```python
from build123d import *

# Parameters (mm, degrees)
SKETCH1_W                  = 84.6
SKETCH1_H                  = 55.3
BOSS_EXTRUDE1_DEPTH        = 2.4
SKETCH2_W                  = 82
SKETCH2_H                  = 54.2
BOSS_EXTRUDE2_DEPTH        = 1.1
SKETCH3_R                  = 0.5
BOSS_EXTRUDE3_DEPTH        = 0.8
CUT_EXTRUDE1_DEPTH         = 1
SKETCH5_W                  = 57
SKETCH5_H                  = 2.4
CUT_EXTRUDE2_DEPTH         = 0.2
SKETCH6_W                  = 45.3
SKETCH6_H                  = 2.4
CUT_EXTRUDE3_DEPTH         = 0.2
SKETCH7_W                  = 44.6
SKETCH7_H                  = 3
BOSS_EXTRUDE4_DEPTH        = 0.15
SKETCH8_W                  = 0.6
SKETCH8_H                  = 12.5
CUT_EXTRUDE4_DEPTH         = 1
SKETCH9_W                  = 4
SKETCH9_H                  = 0.5
BOSS_EXTRUDE5_DEPTH        = 0.2
CHAMFER1_SIZE              = 0.2
CHAMFER1_SIZE_2            = 0.549495484
CHAMFER1_OF_MIRROR4_SIZE   = 0.2
CHAMFER1_OF_MIRROR4_SIZE_2 = 0.549495484
SKETCH10_W                 = 36
SKETCH10_H                 = 1.5
CUT_EXTRUDE5_DEPTH         = 10
BOSS_EXTRUDE7_DEPTH        = 12.5
BOSS_EXTRUDE7_DEPTH_BACK   = 12.5


with BuildPart() as part:
    # Sketch1 → Boss-Extrude1 (new body)
    with BuildSketch(Plane(origin=(0, 0, 0), x_dir=(1, 0, 0), z_dir=(0, 1, 0))):
        Rectangle(SKETCH1_W, SKETCH1_H)
    extrude(amount=-BOSS_EXTRUDE1_DEPTH)

    # Sketch2 → Boss-Extrude2 (add)
    with BuildSketch(Plane(origin=(0, 0, 0), x_dir=(1, 0, 0), z_dir=(0, 1, 0))):
        Rectangle(SKETCH2_W, SKETCH2_H)
    extrude(amount=BOSS_EXTRUDE2_DEPTH)

    # Sketch3 → Boss-Extrude3 (add)
    with BuildSketch(Plane.XZ.offset(2.4)):
        with Locations(Location((-41.8, 27.15, 0), (0, 0, 90))):
            Circle(SKETCH3_R)
        with Locations(Location((41.8, 27.15, 0), (0, 0, 90))):
            Circle(SKETCH3_R)
        with Locations(Location((41.8, -27.15, 0), (0, 0, 270))):
            Circle(SKETCH3_R)
        with Locations(Location((-41.8, -27.15, 0), (0, 0, 270))):
            Circle(SKETCH3_R)
    extrude(amount=BOSS_EXTRUDE3_DEPTH)

    # Sketch4 → Cut-Extrude1 (cut)
    with BuildSketch(Plane.XZ.offset(2.4)):
        with BuildLine():
            Line((-39.7, -22.4), (-41.3, -22.4))
            ThreePointArc((-41.3, -22.4), (-41.724264069, -22.224264069), (-41.9, -21.8))
            Line((-41.9, -21.8), (-41.9, 21.8))
            ThreePointArc((-41.9, 21.8), (-41.724264069, 22.224264069), (-41.3, 22.4))
            Line((-41.3, 22.4), (-39.7, 22.4))
            ThreePointArc((-39.7, 22.4), (-39.275735931, 22.224264069), (-39.1, 21.8))
            Line((-39.1, 21.8), (-39.1, -21.8))
            ThreePointArc((-39.1, -21.8), (-39.275735931, -22.224264069), (-39.7, -22.4))
        make_face()
    extrude(amount=-CUT_EXTRUDE1_DEPTH, mode=Mode.SUBTRACT)

    # Sketch5 → Cut-Extrude2 (cut)
    with BuildSketch(Plane.XY.offset(27.65)):
        with Locations((8.8, -1.2)):
            Rectangle(SKETCH5_W, SKETCH5_H)
    cut_extrude2 = extrude(amount=-CUT_EXTRUDE2_DEPTH, mode=Mode.SUBTRACT)

    # Mirror1: Cut-Extrude2 across plane
    add(cut_extrude2.mirror(Plane.XY), mode=Mode.SUBTRACT)

    # Sketch6 → Cut-Extrude3 (cut)
    with BuildSketch(Plane(origin=(42.3, 0, 0), x_dir=(0, 0, -1), z_dir=(1, 0, 0))):
        with Locations((0, -1.2)):
            Rectangle(SKETCH6_W, SKETCH6_H)
    extrude(amount=-CUT_EXTRUDE3_DEPTH, mode=Mode.SUBTRACT)

    # Sketch7 → Boss-Extrude4 (add)
    with BuildSketch(Plane.XZ.offset(2.4)):
        with Locations((15, 25.85)):
            Rectangle(SKETCH7_W, SKETCH7_H)
    boss_extrude4 = extrude(amount=BOSS_EXTRUDE4_DEPTH)

    # Mirror2: Boss-Extrude4 across plane
    add(boss_extrude4.mirror(Plane.XY))

    # Sketch8 → Cut-Extrude4 (cut)
    with BuildSketch(Plane(origin=(0, 0, 0), x_dir=(1, 0, 0), z_dir=(0, 1, 0))):
        with Locations((41.3, 0)):
            Rectangle(SKETCH8_W, SKETCH8_H)
    extrude(amount=-CUT_EXTRUDE4_DEPTH, mode=Mode.SUBTRACT)

    # Sketch9 → Boss-Extrude5 (add)
    with BuildSketch(Plane.XY.offset(27.45)):
        with Locations((-1.7, -1.2)):
            Rectangle(SKETCH9_W, SKETCH9_H)
        with Locations((26.3, -1.2)):
            Rectangle(SKETCH9_W, SKETCH9_H)
    boss_extrude5 = extrude(amount=BOSS_EXTRUDE5_DEPTH)

    # Chamfer1
    # the kernel refuses this chamfer: 0.549495484, 0.2 mm, written as the material it takes off along each edge
    with BuildSketch(Plane(origin=(29.72549829, -1.45, 27.65), x_dir=(0, -0.0990409022520511, -0.9950833631817485), z_dir=(-1, 0, 0))) as chamfer1_piece_1_section:
        Polygon((CHAMFER1_SIZE * 0.995083363182, -CHAMFER1_SIZE * 0.0990409022521), (-CHAMFER1_SIZE_2 * 0.0990409022324, -CHAMFER1_SIZE_2 * 0.995083362984), (0, 0), align=None)
    chamfer1_piece_1 = extrude(amount=6.85099658, mode=Mode.PRIVATE)
    chamfer1_piece_1 = split(chamfer1_piece_1, bisect_by=Plane(origin=(26.3, -1.261493049, 27.45), z_dir=(0, 0, 1)), keep=Keep.TOP, mode=Mode.PRIVATE)
    add(chamfer1_piece_1, mode=Mode.SUBTRACT)
    with BuildSketch(Plane(origin=(1.72549829, -1.45, 27.65), x_dir=(0, -0.0990409022520511, -0.9950833631817485), z_dir=(-1, 0, 0))) as chamfer1_piece_2_section:
        Polygon((CHAMFER1_SIZE * 0.995083363182, -CHAMFER1_SIZE * 0.0990409022521), (-CHAMFER1_SIZE_2 * 0.0990409022324, -CHAMFER1_SIZE_2 * 0.995083362984), (0, 0), align=None)
    chamfer1_piece_2 = extrude(amount=6.85099658, mode=Mode.PRIVATE)
    chamfer1_piece_2 = split(chamfer1_piece_2, bisect_by=Plane(origin=(-1.7, -1.261493049, 27.45), z_dir=(0, 0, 1)), keep=Keep.TOP, mode=Mode.PRIVATE)
    add(chamfer1_piece_2, mode=Mode.SUBTRACT)

    # Mirror4: Boss-Extrude5 across plane
    add(boss_extrude5.mirror(Plane.XY))

    # Chamfer1 of Mirror4
    # the kernel refuses this chamfer: 0.549495484, 0.2 mm, written as the material it takes off along each edge
    with BuildSketch(Plane(origin=(29.72549829, -1.45, -27.65), x_dir=(0, -0.0990409022520511, 0.9950833631817485), z_dir=(-1, 0, 0))) as chamfer1_of_mirror4_piece_1_section:
        Polygon((CHAMFER1_OF_MIRROR4_SIZE * 0.995083363182, CHAMFER1_OF_MIRROR4_SIZE * 0.0990409022521), (-CHAMFER1_OF_MIRROR4_SIZE_2 * 0.0990409022324, CHAMFER1_OF_MIRROR4_SIZE_2 * 0.995083362984), (0, 0), align=None)
    chamfer1_of_mirror4_piece_1 = extrude(amount=6.85099658, mode=Mode.PRIVATE)
    chamfer1_of_mirror4_piece_1 = split(chamfer1_of_mirror4_piece_1, bisect_by=Plane(origin=(26.3, -1.261493049, -27.45), z_dir=(0, 0, -1)), keep=Keep.TOP, mode=Mode.PRIVATE)
    add(chamfer1_of_mirror4_piece_1, mode=Mode.SUBTRACT)
    with BuildSketch(Plane(origin=(1.72549829, -1.45, -27.65), x_dir=(0, -0.0990409022520511, 0.9950833631817485), z_dir=(-1, 0, 0))) as chamfer1_of_mirror4_piece_2_section:
        Polygon((CHAMFER1_OF_MIRROR4_SIZE * 0.995083363182, CHAMFER1_OF_MIRROR4_SIZE * 0.0990409022521), (-CHAMFER1_OF_MIRROR4_SIZE_2 * 0.0990409022324, CHAMFER1_OF_MIRROR4_SIZE_2 * 0.995083362984), (0, 0), align=None)
    chamfer1_of_mirror4_piece_2 = extrude(amount=6.85099658, mode=Mode.PRIVATE)
    chamfer1_of_mirror4_piece_2 = split(chamfer1_of_mirror4_piece_2, bisect_by=Plane(origin=(-1.7, -1.261493049, -27.45), z_dir=(0, 0, -1)), keep=Keep.TOP, mode=Mode.PRIVATE)
    add(chamfer1_of_mirror4_piece_2, mode=Mode.SUBTRACT)

    # Sketch10 → Cut-Extrude5 (cut)
    with BuildSketch(Plane.ZY.offset(42.3)):
        with Locations((0, -0.75)):
            Rectangle(SKETCH10_W, SKETCH10_H)
    extrude(amount=-CUT_EXTRUDE5_DEPTH, mode=Mode.SUBTRACT)

    # Sketch13 → Boss-Extrude7 (add, two sides: drawn at the far end of the back side and taken through both)
    with BuildSketch(Plane.XY.offset(-BOSS_EXTRUDE7_DEPTH_BACK)):
        with BuildLine():
            Line((-42.05, -0.75), (-32.3, -0.75))
            Line((-32.3, -0.75), (-32.3, -0.65))
            Line((-32.3, -0.65), (-42.058857344, -0.65))
            ThreePointArc((-42.058857344, -0.65), (-42.962715901, -1.720353295), (-42.068005903, -2.798365581))
            Line((-42.068005903, -2.798365581), (-27.318842711, -5.498212402))
            add(Edge.make_bspline(
                [(-27.318842711, -5.498212402), (-27.055971917, -5.550974674), (-26.517605359, -5.672128419), (-25.572291866, -5.932507667), (-24.521729024, -6.300209586), (-23.417642306, -6.772863788), (-22.38181971, -7.248072884), (-21.335698344, -7.694021321), (-20.202294115, -8.077787346), (-19.113789609, -8.318235721), (-18.133663704, -8.446100314), (-17.574099695, -8.487090287), (-17.302374167, -8.5)],
                knots=[6.323e-05, 6.323e-05, 6.323e-05, 6.323e-05, 0.062570215, 0.125077199, 0.250091168, 0.375105137, 0.500119106, 0.625133075, 0.750147043, 0.875161012, 0.937667997, 1.000174981, 1.000174981, 1.000174981, 1.000174981], degree=3))
            Line((-17.302374167, -8.5), (-4.8, -8.5))
            Line((-4.8, -8.5), (-4.8, -8.4))
            Line((-4.8, -8.4), (-17.3, -8.4))
            add(Edge.make_bspline(
                [(-27.3, -5.4), (-22.890715179, -6.284799168), (-21.81761674, -8.185367475), (-17.3, -8.4)],
                knots=[0, 0, 0, 0, 1, 1, 1, 1], degree=3))
            Line((-27.3, -5.4), (-42.05, -2.7))
            ThreePointArc((-42.05, -2.7), (-42.862725794, -1.725), (-42.05, -0.75))
        make_face()
        with BuildLine():
            Line((-32.3, -0.85), (-32.3, -0.75))
            Line((-32.3, -0.75), (-42.05, -0.75))
            ThreePointArc((-42.05, -0.75), (-42.862725794, -1.725), (-42.05, -2.7))
            Line((-42.05, -2.7), (-27.3, -5.4))
            add(Edge.make_bspline(
                [(-27.3, -5.4), (-22.890715179, -6.284799168), (-21.81761674, -8.185367475), (-17.3, -8.4)],
                knots=[0, 0, 0, 0, 1, 1, 1, 1], degree=3))
            Line((-17.3, -8.4), (-4.8, -8.4))
            Line((-4.8, -8.4), (-4.8, -8.3))
            Line((-4.8, -8.3), (-17.297622246, -8.3))
            add(Edge.make_bspline(
                [(-27.281158431, -5.301787389), (-27.015284827, -5.35513952), (-26.470914345, -5.477568661), (-25.513851699, -5.741064097), (-24.450268814, -6.113231913), (-23.336923139, -6.589854571), (-22.30113605, -7.06504573), (-21.26539226, -7.506542017), (-20.151183505, -7.883950719), (-19.082330822, -8.120417996), (-18.117886975, -8.246552851), (-17.565625944, -8.287228528), (-17.297622246, -8.3)],
                knots=[-6.2969e-05, -6.2969e-05, -6.2969e-05, -6.2969e-05, 0.062429979, 0.124922927, 0.249908823, 0.37489472, 0.499880616, 0.624866512, 0.749852409, 0.874838305, 0.937331253, 0.999824201, 0.999824201, 0.999824201, 0.999824201], degree=3))
            Line((-27.281158431, -5.301787389), (-42.031994097, -2.601634419))
            ThreePointArc((-42.031994097, -2.601634419), (-42.762714839, -1.729418922), (-42.040679496, -0.85))
            Line((-42.040679496, -0.85), (-32.3, -0.85))
        make_face()
    extrude(amount=BOSS_EXTRUDE7_DEPTH + BOSS_EXTRUDE7_DEPTH_BACK)


solid = part.part
```
Model file for the job. Use its own axes, mm. A direction names the side the tool comes from. Round coordinates to 2 decimals unless told otherwise and drop trailing zeros. Order: outer loops, then holes, each group sorted by start corner. A loop starts at its lowest first (then second) coordinate and runs counter-clockwise, first axis right, second up. Notation, with made-up numbers: (-31.75, -18) -> (-16.75, -18) arc R18 cw to (-16.75, -11) -> close; hole circle Ø4 at (-34.5, 34.25). An arc over 180 degrees is marked (long way). Use one line per item in the form item = value.
Item 1: Flat gauge pins, fed straight in: pin 1 Ø2.5 at (x, y) = (-15.5, -5.5) entering from -Z; pin 2 Ø0.9 at (x, y) = (-17.5, 1) entering from -Z; pin 3 Ø0.7 at (x, y) = (-5, -1) entering from -Z; pin 4 Ø1.9 at (y, z) = (-1.5, 5.5) entering from +X. Where does each tip first touch, or does it go through?
Returned:
pin_1 = through
pin_2 = -27.1
pin_3 = -27.45
pin_4 = 42.1
Item 2: Cut at A-A, the plane z = 15. Write the cut outline in (x, y).
Returned:
outline = (-42.3, -2.4) -> (-41.9, -2.4) -> (-41.9, -1.5) -> (-42.3, -1.5) -> close; (-41, 0) -> (-32.3, 0) -> (-32.3, -1.5) -> (-39.1, -1.5) -> (-39.1, -2.4) -> (42.1, -2.4) -> (42.1, 0) -> (41, 0) -> (41, 1.1) -> (-41, 1.1) -> close
Item 3: Tool access for faces 1 (the face through (15, -2.55, -26)), 2 (the face through (-1, 1.1, 0)), 3 (the face through (-37, 0, 0)), 4 (the face through (41, 0, 0)): list every direction of +Z, -Z, +X, -X, +Y, -Y with a clear straight run to the whole face (end or side of a thin tool).
Returned:
face_1 = +Z, -Z, -Y
face_2 = +Z, -Z, +X, -X, +Y
face_3 = -X
face_4 = +Y
Item 4: Drill centre lines: line 1 (Y direction, x = -11, z = -10.5); line 2 (X direction, y = -2.25, z = 11.5); line 3 (Y direction, x = -0.5, z = -1). Where is each one in solid material? Low to high.
Returned:
line_1 = -8.5 to -8.3, -2.4 to 1.1
line_2 = -42.83 to -42.59, -42.3 to -41.9, -39.1 to 42.1
line_3 = -2.4 to 1.1
Item 5: Pull direction Y, two halves, no side cores. Call faces 5 (the face through (-40, -1.4, 20)), 6 (the face through (-34.55, -3.97, -0.18)), 7 (the face through (8, -1, -27.45)), 8 (the face through (-11, -8.3, 0)): released by +Y, released by -Y, zero draft, split by the parting line, or undercut.
Returned:
face_5 = released by -Y
face_6 = undercut
face_7 = zero draft
face_8 = undercut
Item 6: Cut at B-B, the plane x = 21.5. Write the cut outline in (y, z), and give its area (3 significant figures).
Returned:
outline = (-2.55, -27.35) -> (-2.4, -27.35) -> (-2.4, -27.45) -> (0, -27.45) -> (0, -27.1) -> (1.1, -27.1) -> (1.1, 27.1) -> (0, 27.1) -> (0, 27.45) -> (-2.4, 27.45) -> (-2.4, 27.35) -> (-2.55, 27.35) -> (-2.55, 24.35) -> (-2.4, 24.35) -> (-2.4, -24.35) -> (-2.55, -24.35) -> close
area = 192 mm^2
